```python
from build123d import *

# Parameters (mm, degrees)
SKETCH_1_W           = 35
SKETCH_1_H           = 35
SKETCH_1_R           = 12.7
EXTRUDE_1_DEPTH      = 3
EXTRUDE_2_DEPTH      = 2
EXTRUDE_2_DEPTH_BACK = 5
SKETCH_2_R           = 2
SKETCH_3_R           = 4
EXTRUDE_3_DEPTH      = 4
EXTRUDE_START        = 3
SKETCH_4_W           = 35
SKETCH_4_H           = 35
SKETCH_4_R           = 12.7
EXTRUDE_4_DEPTH      = 3
SKETCH_5_W           = 51.816122842
SKETCH_5_H           = 54.036228948
CUT_EXTRUDE_1_DEPTH  = 3
SKETCH_7_W           = 35
SKETCH_7_H           = 35
CUT_EXTRUDE_3_DEPTH  = 3
FILLET_1_R           = 2


with BuildPart() as part:
    # 草图1 → 凸台-拉伸1 (new body)
    with BuildSketch(Plane.XY):
        Rectangle(SKETCH_1_W, SKETCH_1_H)
        Circle(SKETCH_1_R, mode=Mode.SUBTRACT)
    extrude(amount=EXTRUDE_1_DEPTH)

    # 草图2 → 凸台-拉伸2 (add, two sides: drawn at the far end of the back side and taken through both)
    with BuildSketch(Plane.XY.offset(3).offset(-EXTRUDE_2_DEPTH_BACK)):
        with Locations((-12.196699141, 12.196699141)):
            Circle(SKETCH_2_R)
        with Locations((12.196699141, -12.196699141)):
            Circle(SKETCH_2_R)
        with Locations((-12.196699141, -12.196699141)):
            Circle(SKETCH_2_R)
    extrude(amount=EXTRUDE_2_DEPTH + EXTRUDE_2_DEPTH_BACK)

    # 草图3 → 凸台-拉伸3 (add)
    with BuildSketch(Plane.XY.offset(5)):
        with Locations((-12.196699141, 12.196699141)):
            Circle(SKETCH_3_R)
        with Locations((-12.196699141, -12.196699141)):
            Circle(SKETCH_3_R)
        with Locations((12.196699141, -12.196699141)):
            Circle(SKETCH_3_R)
    extrude(amount=EXTRUDE_3_DEPTH)

    # 草图4 → 凸台-拉伸4 (add)
    with BuildSketch(Plane(origin=(0, 0, -2), x_dir=(-1, 0, 0), z_dir=(0, 0, -1)).offset(EXTRUDE_START)):
        Rectangle(SKETCH_4_W, SKETCH_4_H)
        with Locations(Location((0, 0, 0), (0, 0, 180))):
            Circle(SKETCH_4_R, mode=Mode.SUBTRACT)
    extrude(amount=-EXTRUDE_4_DEPTH)

    # 草图5 → 切除-拉伸1 (cut)
    with BuildSketch(Plane.XY.offset(3)):
        with Locations((17.5, 17.5)):
            Rectangle(SKETCH_5_W, SKETCH_5_H)
    extrude(amount=-CUT_EXTRUDE_1_DEPTH, mode=Mode.SUBTRACT)

    # 草图7 → 切除-拉伸3 (cut)
    with BuildSketch(Plane(origin=(0, 0, -5), x_dir=(-1, 0, 0), z_dir=(0, 0, -1))):
        with Locations((-17.5, 17.5)):
            Rectangle(SKETCH_7_W, SKETCH_7_H)
    extrude(amount=-CUT_EXTRUDE_3_DEPTH, mode=Mode.SUBTRACT)

    # 圆角1
    fillet_1_edges = [part.edges().sort_by_distance(p)[0] for p in [
        (8.408061421, -9.518114474, 1.5),
        (-8.408061421, 9.518114474, 1.5),
        (-8.408061421, 17.5, 1.5),
        (17.5, -9.518114474, 1.5),
        (0, 17.5, -3.5),
        (17.5, 0, -3.5),
    ]]
    fillet(fillet_1_edges, radius=FILLET_1_R)


solid = part.part
```
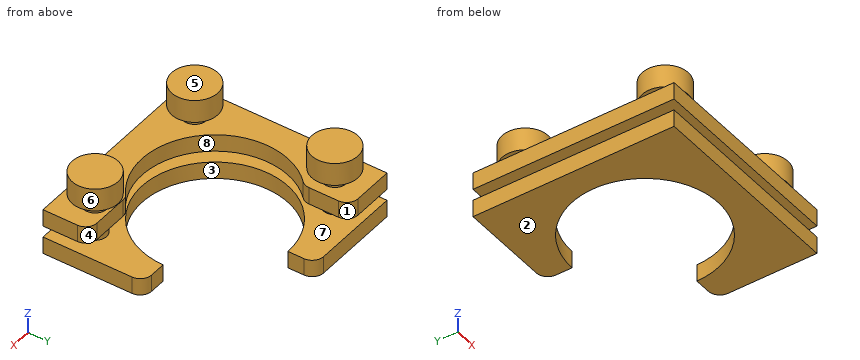
The listing builds one solid part. Answer for the finished solid, in the listing's coordinates (mm). Face numbers are marked on the shaded views. A direction names the side the tool comes from. Round coordinates to 2 decimals unless told otherwise and drop trailing zeros. Write each loop counter-clockwise with the first axis right and the second up, starting at its lowest first coordinate (ties: lowest second). Pieces come first, ordered by that corner, then holes. Notation, with made-up numbers: (7, 80.5) -> (21, 80.5) arc R26 ccw to (21, 115.5) -> close; hole circle Ø11 at (47, 70.25). An arc over 180 degrees is marked (long way). Use CSV: the item, a comma, the result in double quotes. Start each with the question number.
(1) Section D-D on y = -6 is taken. Give the vertices of the cut face in (x, z), then the cut area to 3 significant figures.
(2) The mould has two halves that part along Y. Classify the marked faces 1, 2 and 3: released by +Y, released by -Y, zero draft, split by the parting line, or undercut.
(3) Each of these flat-tipped pins is pushed along its axis until it touches: pin 1 (17.5 mm diameter, centred on x = 4.5, y = 0, fed in from +Z); pin 2 (0.9 mm diameter, centred on x = 11, z = 2, fed in from +Y); pin 3 (2 mm diameter, centred on x = 14, z = 5.5, fed in from -Y). Where does it stop, or does it pass through?
(4) Section A-A on z = -2.5 is taken. Give the vertices of the cut face in (x, y).
(5) Section C-C on x = 5 is taken. Give the vertices of the cut face in (y, z), then the cut area to 3 significant figures.
(6) Section B-B on y = 2 is taken. Give the vertices of the cut face in (x, z), then the cut area to 3 significant figures.
(7) Which of the six approach directions +Z, -Z, +X, -X, +Y, -Y give full straight-line access (tool end or side, diameter ignored) to the marked faces 4, 5, 6, 7 and 8?
(8) Consider L1, parallel to Z at x = -13.5, y = 10.5; L2, parallel to Z at x = 3, y = -15; L3, parallel to Y at x = 15, z = -3.5. Determine where each line is inside the solid, lowest interval first. Write a range as from..to.
A:
1,outline,"(-17.5, -5) -> (-11.19, -5) -> (-11.19, -2) -> (-17.5, -2) -> close; (-17.5, 0) -> (-11.19, 0) -> (-11.19, 3) -> (-17.5, 3) -> close; (11.19, -5) -> (17.5, -5) -> (17.5, -2) -> (11.19, -2) -> close"
1,area,"56.8 mm²"
2,face 1,"released by +Y"
2,face 2,"zero draft"
2,face 3,"undercut"
3,pin 1,"stops at z = -2"
3,pin 2,"stops at y = -9.52"
3,pin 3,"stops at y = -16.12"
4,outline,"(-17.5, -17.5) -> (17.5, -17.5) -> (17.5, -2) arc R2 ccw to (15.5, 0) -> (12.7, 0) arc R12.7 cw (long way) to (0, 12.7) -> (0, 15.5) arc R2 ccw to (-2, 17.5) -> (-17.5, 17.5) -> close"
5,outline,"(-17.5, -5) -> (-11.67, -5) -> (-11.67, -2) -> (-17.5, -2) -> close; (-17.5, 0) -> (-11.67, 0) -> (-11.67, 3) -> (-17.5, 3) -> close"
5,area,"35.0 mm²"
6,outline,"(-17.5, -5) -> (-12.54, -5) -> (-12.54, -2) -> (-17.5, -2) -> close; (-17.5, 0) -> (-12.54, 0) -> (-12.54, 3) -> (-17.5, 3) -> close"
6,area,"29.8 mm²"
7,face 4,"+Z, +X, +Y"
7,face 5,"+Z, +X, -X, +Y, -Y"
7,face 6,"+Z"
7,face 7,"none"
7,face 8,"+Z, -Z"
8,L1,"z = -5..-2, 0..3, 5..9"
8,L2,"z = -5..-2, 0..3"
8,L3,"y = -17.5..0"
